Design review of the part built by this model. Coordinates are the model's own, in mm. Face numbers are marked on the shaded views. A direction names the side the tool comes from. Coordinates: 2 decimals unless noted, no trailing zeros. Order: outer loops, then holes, each group sorted by start corner. A loop starts at its lowest first (then second) coordinate and runs counter-clockwise, first axis right, second up. Notation, with made-up numbers: M 79,24 L 124,24 A20 ccw 124,29 Z; hole C 63.25,-35 d2. An arc over 180 degrees is marked long. Answer as a JSON object with one key per item and string values.
from build123d import *

# Parameters (mm, degrees)
SKETCH2_R           = 2.55
SKETCH2_W           = 30
SKETCH2_H           = 15
BOSS_EXTRUDE1_DEPTH = 35
SKETCH3_R           = 4.3
CUT_EXTRUDE1_DEPTH  = 29.6
SKETCH4_R           = 4.3
CUT_EXTRUDE2_DEPTH  = 29.6
SKETCH5_R           = 2.55
CUT_EXTRUDE3_DEPTH  = 29.6
FILLET1_R           = 5
CHAMFER1_SIZE       = 1


with BuildPart() as part:
    # Sketch2 → Boss-Extrude1 (new body)
    # profile 1 of 2: a face of its own
    with BuildSketch(Plane.XY):
        Polygon((-326.5, 320), (-311.5, 320), (-311.5, 345), (-311.5, 360), (-326.5, 360), align=None)
        with Locations((-319, 327)):
            Circle(SKETCH2_R, mode=Mode.SUBTRACT)
        with Locations((-319, 352.5)):
            Circle(SKETCH2_R, mode=Mode.SUBTRACT)
    # profile 2 of 2: a face of its own
    with BuildSketch(Plane.XY):
        with Locations((-296.5, 352.5)):
            Rectangle(SKETCH2_W, SKETCH2_H)
        with Locations((-288.5, 352.5)):
            Circle(SKETCH2_R, mode=Mode.SUBTRACT)
    extrude(amount=BOSS_EXTRUDE1_DEPTH)

    # Sketch3 → Cut-Extrude1 (cut)
    with BuildSketch(Plane.XY.offset(35)):
        with Locations((-319, 352.5)):
            Circle(SKETCH3_R)
        with Locations((-319, 327)):
            Circle(SKETCH3_R)
        with Locations((-288.5, 352.5)):
            Circle(SKETCH3_R)
    extrude(amount=-CUT_EXTRUDE1_DEPTH, mode=Mode.SUBTRACT)

    # Sketch4 → Cut-Extrude2 (cut)
    with BuildSketch(Plane(origin=(0, 0, 0), x_dir=(-1, 0, 0), z_dir=(0, 0, -1))):
        with Locations((303.5, 352.5)):
            Circle(SKETCH4_R)
    extrude(amount=-CUT_EXTRUDE2_DEPTH, mode=Mode.SUBTRACT)

    # Sketch5 → Cut-Extrude3 (cut)
    with BuildSketch(Plane(origin=(0, 0, 29.6), x_dir=(-1, 0, 0), z_dir=(0, 0, -1))):
        with Locations((303.5, 352.5)):
            Circle(SKETCH5_R)
    extrude(amount=-CUT_EXTRUDE3_DEPTH, mode=Mode.SUBTRACT)

    # Fillet1
    fillet1_edges = [part.edges().sort_by_distance(p)[0] for p in [
        (-311.5, 345, 17.5),
        (-281.5, 345, 17.5),
        (-281.5, 360, 17.5),
        (-311.5, 320, 17.5),
        (-326.5, 320, 17.5),
        (-326.5, 360, 17.5),
    ]]
    fillet(fillet1_edges, radius=FILLET1_R)

    # Chamfer1
    chamfer1_edges = [part.edges().sort_by_distance(p)[0] for p in [
        (-292.8, 352.5, 35),
        (-323.3, 327, 35),
        (-323.3, 352.5, 35),
        (-299.2, 352.5, 0),
    ]]
    chamfer(chamfer1_edges, length=CHAMFER1_SIZE)


solid = part.part
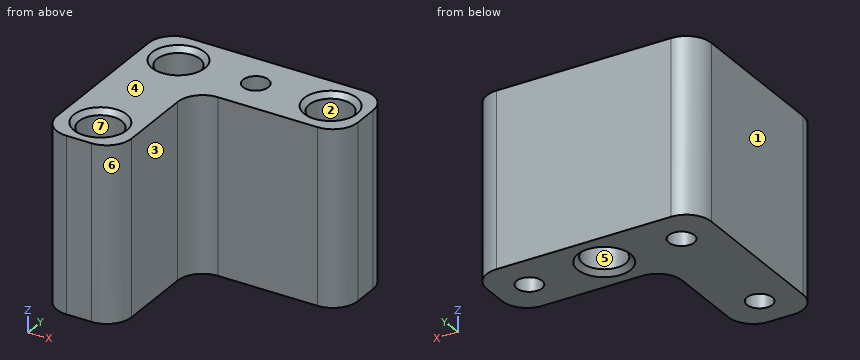
1) Add section C-C (x = -288.5). State the section outline as (y, z) points.
Taken from the geometry:
{"outline": "M 345,0 L 349.95,0 L 349.95,5.4 L 348.2,5.4 L 348.2,34 L 347.2,35 L 345,35 Z; M 355.05,0 L 360,0 L 360,35 L 357.8,35 L 356.8,34 L 356.8,5.4 L 355.05,5.4 Z"}
2) Add section D-D (z = 18). State the section outline as (x, y) points.
Taken from the geometry:
{"outline": "M -326.5,325 A5 ccw -321.5,320 L -316.5,320 A5 ccw -311.5,325 L -311.5,340 A5 cw -306.5,345 L -286.5,345 A5 ccw -281.5,350 L -281.5,355 A5 ccw -286.5,360 L -321.5,360 A5 ccw -326.5,355 Z; hole C -319,327 d8.6; hole C -319,352.5 d8.6; hole C -303.5,352.5 d8.6; hole C -288.5,352.5 d8.6"}
3) Add section A-A (x = -319). State the section outline as (y, z) points.
Taken from the geometry:
{"outline": "M 320,0 L 324.45,0 L 324.45,5.4 L 322.7,5.4 L 322.7,34 L 321.7,35 L 320,35 Z; M 329.55,0 L 349.95,0 L 349.95,5.4 L 348.2,5.4 L 348.2,34 L 347.2,35 L 332.3,35 L 331.3,34 L 331.3,5.4 L 329.55,5.4 Z; M 355.05,0 L 360,0 L 360,35 L 357.8,35 L 356.8,34 L 356.8,5.4 L 355.05,5.4 Z"}
4) Add section B-B (y = 327). State the section outline as (x, z) points.
Taken from the geometry:
{"outline": "M -326.5,0 L -321.55,0 L -321.55,5.4 L -323.3,5.4 L -323.3,34 L -324.3,35 L -326.5,35 Z; M -316.45,0 L -311.5,0 L -311.5,35 L -313.7,35 L -314.7,34 L -314.7,5.4 L -316.45,5.4 Z"}
5) Insertion check: pin 1 Ø6 at (y, z) = (330, 14.5) entering from +X; pin 2 Ø7.5 at (x, y) = (-288.5, 352.5) entering from +Z; pin 3 Ø4.5 at (x, y) = (-288.5, 352.5) entering from +Z; pin 4 Ø1 at (x, z) = (-293.5, 20) entering from -Y. Each pin has a flat end and moves straight along its axis. Give the tip position at first contact, or say it passes through.
Taken from the geometry:
{"pin 1": "stops at x = -311.5", "pin 2": "stops at z = 5.4", "pin 3": "passes through", "pin 4": "stops at y = 345"}
6) Tool access review of the marked faces 1, 2 and 3: name each direction out of +Z, -Z, +X, -X, +Y, -Y from which nothing blocks a thin tool from reaching the whole face with its end or side.
Taken from the geometry:
{"face 1": "+Z, -Z, -X, +Y, -Y", "face 2": "+Z", "face 3": "+Z, -Z, +X, -Y"}
7) To check wall thickness, follow L1, parallel to X at y = 352.5, z = 12.25; L2, parallel to Y at x = -318, z = 20; L3, parallel to Y at x = -288.5, z = 4.1. State the ranges of each line that lie inside material, in increasing order.
Taken from the geometry:
{"L1": "x = -326.5 to -323.3, -314.7 to -307.8, -299.2 to -292.8, -284.2 to -281.5", "L2": "y = 320 to 322.82, 331.18 to 348.32, 356.68 to 360", "L3": "y = 345 to 349.95, 355.05 to 360"}
8) Mouldability with a two-part tool opening along X and no side actions: class the marked faces 4, 5, 6 and 7 as released by +X, released by -X, zero draft, split by the parting line, or undercut.
Taken from the geometry:
{"face 4": "zero draft", "face 5": "undercut", "face 6": "released by +X", "face 7": "undercut"}
